Part model, mm, in its own coordinate system. Round coordinates to 2 decimals unless told otherwise and drop trailing zeros. Loops run counter-clockwise (first coordinate to the right, second up) from the corner with the lowest first, then second, coordinate; pieces in that order, holes last.
from build123d import *

# Parameters (mm, degrees)
SKETCH_2_R          = 7
EXTRUDE_1_DEPTH     = 100
CUT_EXTRUDE_3_DEPTH = 8
SKETCH_6_R          = 11
CUT_EXTRUDE_5_DEPTH = 3.55
SKETCH_5_R          = 4.01
CUT_EXTRUDE_6_DEPTH = 80


with BuildPart() as part:
    # 草图2 → 凸台-拉伸1 (new body)
    with BuildSketch(Plane.XY):
        Circle(SKETCH_2_R)
    extrude(amount=EXTRUDE_1_DEPTH)

    # 草图3 → 切除-拉伸3 (cut, symmetric)
    with BuildSketch(Plane(origin=(0, 0, 0), x_dir=(1, 0, 0), z_dir=(0, 1, 0))):
        with BuildLine():
            ThreePointArc((-7, -7), (0, 0), (7, -7))
            Line((7, -7), (17.530133207, -7))
            ThreePointArc((17.530133207, -7), (0, 10.530133207), (-17.530133207, -7))
            Line((-17.530133207, -7), (-7, -7))
        make_face()
    extrude(amount=CUT_EXTRUDE_3_DEPTH, both=True, mode=Mode.SUBTRACT)

    # 草图6 → 切除-拉伸5 (cut, symmetric)
    with BuildSketch(Plane(origin=(0, 0, 0), x_dir=(1, 0, 0), z_dir=(0, 1, 0))):
        with Locations((0, -7)):
            Circle(SKETCH_6_R)
    extrude(amount=CUT_EXTRUDE_5_DEPTH, both=True, mode=Mode.SUBTRACT)

    # 草图5 → 切除-拉伸6 (cut, symmetric)
    with BuildSketch(Plane(origin=(0, 0, 0), x_dir=(1, 0, 0), z_dir=(0, 1, 0))):
        with Locations(Location((0, -7, 0), (0, 0, 270))):
            Circle(SKETCH_5_R)
    extrude(amount=CUT_EXTRUDE_6_DEPTH, both=True, mode=Mode.SUBTRACT)


solid = part.part
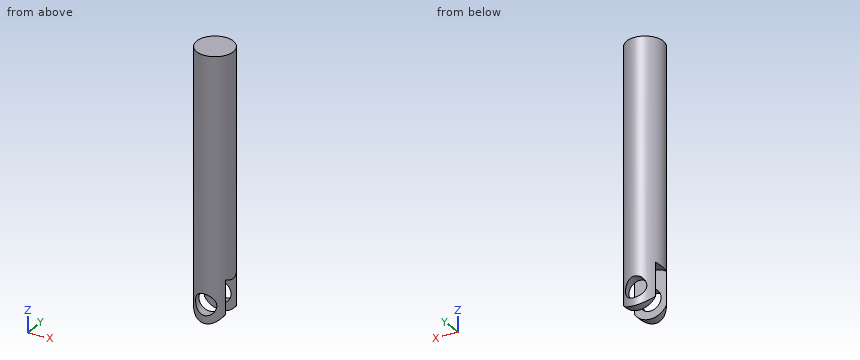
1) Slice it at A-A, the plane x = 0. Give the cut face in (y, z).
Values:
outline: (-7, 0) - (-3.55, 0) - (-3.55, 2.99) - (-7, 2.99) - close; (-7, 11.01) - (-3.55, 11.01) - (-3.55, 18) - (3.55, 18) - (3.55, 11.01) - (7, 11.01) - (7, 100) - (-7, 100) - close; (3.55, 0) - (7, 0) - (7, 2.99) - (3.55, 2.99) - close
2) Slice it at B-B, the plane z = 7. Give the cut face in (x, y), then the cut area to 3 significant figures.
Values:
outline: (-6.03, -3.55) arc R7 ccw to (-4.01, -5.74) - (-4.01, -3.55) - close; (-6.03, 3.55) - (-4.01, 3.55) - (-4.01, 5.74) arc R7 ccw to start; (4.01, -5.74) arc R7 ccw to (6.03, -3.55) - (4.01, -3.55) - close; (4.01, 3.55) - (6.03, 3.55) arc R7 ccw to (4.01, 5.74) - close
area: 10.1 mm2
3) Drop flat-ended pins along their axis: pin 1 Ø3.5 at (x, z) = (-2.5, 6) entering from -Y; pin 2 Ø6 at (x, z) = (-2, 7.5) entering from +Y; pin 3 Ø2 at (x, z) = (4.5, 25) entering from -Y; pin 4 Ø6 at (x, z) = (-1, 70.5) entering from -Y. Give the stop position or say it passes through.
Values:
pin 1: stops at y = -6.33
pin 2: stops at y = 6.72
pin 3: stops at y = -6.06
pin 4: stops at y = -7
4) Slice it at D-D, the plane x = 5. Give the cut face in (y, z).
Values:
outline: (-4.9, 2.1) - (-3.55, 2.1) - (-3.55, 16.8) - (3.55, 16.8) - (3.55, 2.1) - (4.9, 2.1) - (4.9, 100) - (-4.9, 100) - close
5) Slice it at C-C, the plane y = -5.25. Give the cut face in (x, z).
Values:
outline: (-4.63, 1.75) arc R7 ccw to (4.63, 1.75) - (4.63, 100) - (-4.63, 100) - close; hole circle Ø8.02 at (0, 7)
6) Wall check: line 1 along Z through (x, y) = (0, 5.6); line 2 along Y through (x, z) = (-0.25, 20); line 3 along Y through (x, z) = (-3.75, 12). Give the ranges that are in metal, low to high.
Values:
line 1: z = 0 to 2.99, 11.01 to 100
line 2: y = -7 to 7
line 3: y = -5.91 to -3.55, 3.55 to 5.91
